Here's how the part is built. I have some questions about the finished solid (model axes, mm). A direction names the side the tool comes from. Round coordinates to 2 decimals unless told otherwise and drop trailing zeros. Write each loop counter-clockwise with the first axis right and the second up, starting at its lowest first coordinate (ties: lowest second). Pieces come first, ordered by that corner, then holes. Notation, with made-up numbers: (50, 29.5) -> (79, 29.5) arc R30 ccw to (79, 54.5) -> close; hole circle Ø8 at (87, -31). An arc over 180 degrees is marked (long way). Answer as CSV lines item,"result".
```python
from build123d import *

# Parameters (mm, degrees)
SKETCH1_W           = 35
SKETCH1_H           = 120
BOSS_EXTRUDE1_DEPTH = 70
SKETCH2_R           = 32.5
BOSS_EXTRUDE2_DEPTH = 80
SKETCH3_R           = 3.175
CUT_EXTRUDE1_DEPTH  = 10


with BuildPart() as part:
    # Sketch1 → Boss-Extrude1 (new body)
    with BuildSketch(Plane(origin=(0, 0, 0), x_dir=(1, 0, 0), z_dir=(0, 1, 0))):
        with Locations((17.5, 60)):
            Rectangle(SKETCH1_W, SKETCH1_H)
    extrude(amount=BOSS_EXTRUDE1_DEPTH)

    # Sketch2 → Boss-Extrude2 (add)
    with BuildSketch(Plane.ZY):
        with Locations((-60.174932569, 34.890792619)):
            Circle(SKETCH2_R)
    extrude(amount=BOSS_EXTRUDE2_DEPTH)

    # Sketch3 → Cut-Extrude1 (cut)
    with BuildSketch(Plane.XZ):
        with Locations(Location((17.432872718, -60.623445189, 0), (0, 0, 270))):
            Circle(SKETCH3_R)
    extrude(amount=-CUT_EXTRUDE1_DEPTH, mode=Mode.SUBTRACT)


solid = part.part
```
1. Suppose I cut it at A-A on y = 43. Please give me the cut outline in (x, z).
Numbers:
outline,"(-80, -91.65) -> (0, -91.65) -> (0, -120) -> (35, -120) -> (35, 0) -> (0, 0) -> (0, -28.7) -> (-80, -28.7) -> close"
2. Suppose I cut it at D-D on x = -9. Please give me the cut outline in (y, z).
Numbers:
outline,"circle Ø65 at (34.89, -60.17)"
3. Suppose I cut it at B-B on z = -82.5. Please give me the cut outline in (x, y), and give its area (3 significant figures).
Numbers:
outline,"(-80, 11.27) -> (0, 11.27) -> (0, 0) -> (35, 0) -> (35, 70) -> (0, 70) -> (0, 58.51) -> (-80, 58.51) -> close"
area,"6,230 mm^2"
4. Suppose I cut it at C-C on z = -14. Please give me the cut outline in (x, y), and give its area (3 significant figures).
Numbers:
outline,"(0, 0) -> (35, 0) -> (35, 70) -> (0, 70) -> close"
area,"2,450 mm^2"
5. If we mould it in two halves opening along Z, with no side actions, what happens to faces 4 (the face through (17, 10, -61)), 5 (the face through (-39.44, 44.653, -29.176)), 6 (the face through (17, 35, 0))? For each: released by +Z, released by -Z, zero draft, split by the parting line, or undercut.
Numbers:
face 4,"undercut"
face 5,"split by the parting line"
face 6,"released by +Z"
6. On a 3-axis mill with a long thin cutter (end or side, diameter ignored), from which of +Z, -Z, +X, -X, +Y, -Y can I reach the whole of each face in a straight line? I mean faces 1 (the face through (0, 66, -72)), 2 (the face through (17.57, 4.93, -57.45)), 3 (the face through (21, 0, -61)). Say none if no direction works.
Numbers:
face 1,"-X"
face 2,"-Y"
face 3,"+Z, -Z, +X, -X, -Y"
7. For pin 1 Ø3 at (x, z) = (-60, -87.5) entering from -Y; pin 2 Ø5 at (x, z) = (17.43, -60.62) entering from -Y; pin 3 Ø1.5 at (x, z) = (-30.5, -47) entering from -Y; pin 4 Ø2 at (x, z) = (-55.5, -95) entering from -Y, each with a flat end and sliding along its axis, tell me the tip position at first contact or that it passes through.
Numbers:
pin 1,"stops at y = 15.16"
pin 2,"stops at y = 10"
pin 3,"stops at y = 4.86"
pin 4,"passes through"
8. If I drill on line 1 (X direction, y = 4, z = -82); line 2 (Y direction, x = -72.5, z = -59); line 3 (Z direction, x = -34, y = 63.5), over which ranges is the centre line in solid material (lowest first)?
Numbers:
line 1,"x = 0 to 35"
line 2,"y = 2.41 to 67.37"
line 3,"z = -75.59 to -44.76"
